The model under review builds one solid part; all positions refer to its coordinate system, in mm. Coordinates: 2 decimals unless noted, no trailing zeros. Order: outer loops, then holes, each group sorted by start corner. A loop starts at its lowest first (then second) coordinate and runs counter-clockwise, first axis right, second up. Notation, with made-up numbers: M 33.25,56.5 L 80.25,56.5 A24 ccw 80.25,79.5 Z; hole C 45,-11 d5. An arc over 180 degrees is marked long. One line per item, written item: value.
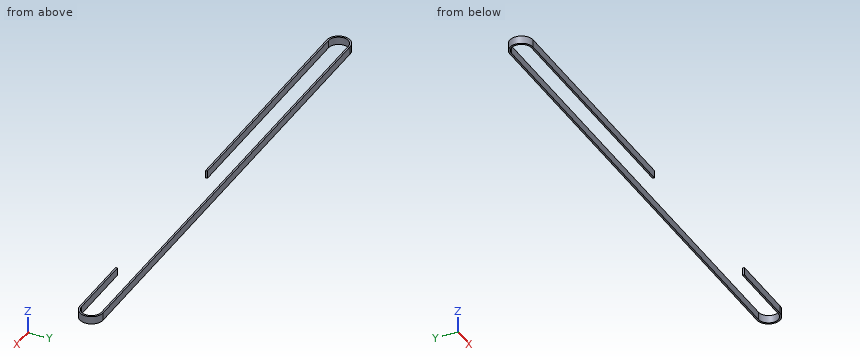
Autodesk Inventor part; units mm, degrees
ref_plane "YZ Plane" through (0, 0, 0) normal (1, 0, 0) x (0, 1, 0)
ref_plane "XZ Plane" through (0, 0, 0) normal (0, 1, 0) x (-1, 0, 0)
ref_plane "XY Plane" through (0, 0, 0) normal (0, 0, 1) x (1, 0, 0)
sketch "Skizze1" plane through (0, 0, 0) normal (0, 0, 1) x (1, 0, 0)
  circle A0 centre (-380.0469, -116.0198) radius 3 construction
  circle A1 centre (-10.0469, -116.0198) radius 3.1 construction
  circle A2 centre (-380.0469, -116.0198) radius 9.05 construction
  circle A3 centre (-10.0469, -116.0198) radius 9.05 construction
  line L0 (-10.0469, -106.9698) -> (-380.0469, -106.9698)
  line L1 (-380.0469, -116.0198) -> (-380.0469, -106.9698) construction
  arc A4 (-380.0469, -106.9698) -> (-380.0469, -125.0698) centre (-380.0469, -116.0198) ccw
  line L2 (-380.0469, -125.0698) -> (-10.0469, -125.0698)
  arc A5 (-10.0469, -125.0698) -> (-10.0469, -106.9698) centre (-10.0469, -116.0198) ccw
  circle A6 centre (-380.0469, -116.0198) radius 7.65 construction
  circle A7 centre (-10.0469, -116.0198) radius 7.65 construction
  line L3 (-10.0469, -123.6698) -> (-380.0469, -123.6698)
  arc A8 (-380.0469, -108.3698) -> (-380.0469, -123.6698) centre (-380.0469, -116.0198) ccw
  line L4 (-380.0469, -108.3698) -> (-10.0469, -108.3698)
  arc A9 (-10.0469, -123.6698) -> (-10.0469, -108.3698) centre (-10.0469, -116.0198) ccw
  line L5 (-198.5469, -125.0698) -> (-198.5469, -123.6698)
  line L6 (-63.6869, -123.6698) -> (-63.6869, -125.0698)
  line L7 (-10.0469, -124.2698) -> (-380.0469, -124.2698) construction
  arc A10 (-380.0469, -107.7698) -> (-380.0469, -124.2698) centre (-380.0469, -116.0198) ccw construction
  line L8 (-380.0469, -107.7698) -> (-10.0469, -107.7698) construction
  arc A11 (-10.0469, -124.2698) -> (-10.0469, -107.7698) centre (-10.0469, -116.0198) ccw construction
  point P0 (0, 0)
  dimension "d0" = 370
  dimension "d3" = 370
  dimension "d8" = 53.64
  dimension "d9" = 181.5
  dimension "d11" = 181.5
  dimension "d12" = 370
  dimension "d13" = 53.64
  dimension "d14" = 8.25
  dimension "d15" = 8.25
  dimension "d16" = 15.3
  dimension "d17" = 15.3
  dimension "d18" = 0.8
  dimension "d19" = 1.4
  dimension "d20" = 18.1
extrude "Extrusion1" add sketch "Skizze1" along normal mid plane 6 contours A5 L2 L6 L3 A9 L4 A8 L5 A4 L0
equation "\"d8\" = Riemen_L_UpBottom"
equation "\"d9\" = Riemen_L_BottomUp"
equation "\"d17\" = d16"
equation "\"d2\" = d1"
equation "\"Riemen_L_UpBottom\" = 53.64"
equation "\"Bogenlaenge\" = 27.70885"
equation "\"Riemenlaenge\" = d12 + 2 * Bogenlaenge + d13 + d11"
equation "\"Riemen_L_BottomUp\" = 181.5"
properties part number "Riemen_T5" material "Gummi"
(1) Insertion check: pin 1 Ø1.5 at (y, z) = (-124.5, -1) entering from +X; pin 2 Ø1.5 at (y, z) = (-114, -2) entering from -X; pin 3 Ø1 at (y, z) = (-122, 1.5) entering from +X; pin 4 Ø10 at (x, y) = (-225, -110.5) entering from -Z. Each pin has a flat end and moves straight along its axis. Give the tip position at first contact, or say it passes through.
Geometry results:
pin 1: stops at x = -5.34
pin 2: stops at x = -389.01
pin 3: stops at x = -2.84
pin 4: stops at z = -3
(2) For L1, parallel to Y at x = -370, z = 0.4; L2, parallel to X at y = -116.25, z = -1.6; L3, parallel to Y at x = -88, z = 2.45, list the stretches that pass through material, from the lowest coordinate up.
Geometry results:
L1: y = -125.07 to -123.67, -108.37 to -106.97
L2: x = -389.09 to -387.69, -2.4 to -1
L3: y = -108.37 to -106.97
(3) We need section C-C, the plane y = -119. State the section outline as (x, z) points.
Geometry results:
outline: M -388.59,-3 L -387.09,-3 L -387.09,3 L -388.59,3 Z; M -3,-3 L -1.5,-3 L -1.5,3 L -3,3 Z
(4) We need section D-D, the plane x = -128.5. State the section outline as (y, z) points, plus the area to 3 significant figures.
Geometry results:
outline: M -108.37,-3 L -106.97,-3 L -106.97,3 L -108.37,3 Z
area: 8.40 mm2
(5) We need section A-A, the plane x = -363. State the section outline as (y, z) points, plus the area to 3 significant figures.
Geometry results:
outline: M -125.07,-3 L -123.67,-3 L -123.67,3 L -125.07,3 Z; M -108.37,-3 L -106.97,-3 L -106.97,3 L -108.37,3 Z
area: 16.8 mm2
(6) We need section B-B, the plane z = -1.05. State the section outline as (x, y) points.
Geometry results:
outline: M -380.05,-125.07 L -198.55,-125.07 L -198.55,-123.67 L -380.05,-123.67 A7.65 cw -380.05,-108.37 L -10.05,-108.37 A7.65 cw -10.05,-123.67 L -63.69,-123.67 L -63.69,-125.07 L -10.05,-125.07 A9.05 ccw -10.05,-106.97 L -380.05,-106.97 A9.05 ccw Z
